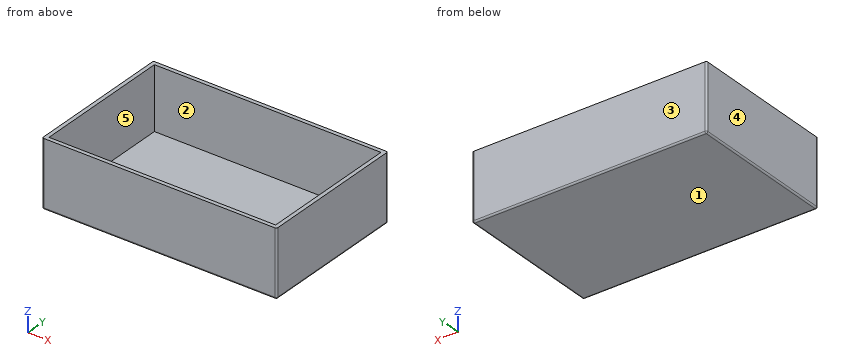
Autodesk Inventor part; units mm, degrees
ref_plane "YZ Plane" through (0, 0, 0) normal (1, 0, 0) x (0, 1, 0)
ref_plane "XZ Plane" through (0, 0, 0) normal (0, 1, 0) x (-1, 0, 0)
ref_plane "XY Plane" through (0, 0, 0) normal (0, 0, 1) x (1, 0, 0)
sketch "Sketch3" plane through (0, 0, 0) normal (0, 0, 1) x (1, 0, 0)
  line L0 (0, -133) -> (0, 133)
  line L1 (-210, 0) -> (210, 0)
  line L2 (-150, -95) -> (150, -95)
  line L3 (150, -95) -> (150, 95)
  line L4 (150, 95) -> (-150, 95)
  line L5 (-150, 95) -> (-150, -95)
  line L6 (-150, -95) -> (150, 95) construction
  line L7 (150, -95) -> (-150, 95) construction
  line L8 (-145, -90) -> (145, -90)
  line L9 (145, -90) -> (145, 90)
  line L10 (145, 90) -> (-145, 90)
  line L11 (-145, 90) -> (-145, -90)
  line L12 (-145, -90) -> (145, 90) construction
  line L13 (145, -90) -> (-145, 90) construction
  point P0 (0, 0)
  dimension "d0" = 300
  dimension "d1" = 190
  dimension "d2" = 290
  dimension "d3" = 180
extrude "Extrusion1" add sketch "Sketch3" along normal blind 85 contours L2 L5 L1 L11 L8 L0 | L0 L8 L9 L1 L3 L2 | L5 L4 L0 L10 L11 L1 | L1 L9 L10 L0 L4 L3
extrude "Extrusion2" add sketch "Sketch3" along normal blind 5 contours L8 L11 L1 L0 | L0 L1 L9 L8 | L1 L11 L10 L0 | L0 L10 L9 L1
fillet "Fillet1" radius 2 8 edges at (150, -95, 42.5) (150, 95, 42.5) (-150, 95, 42.5) (-150, -95, 42.5) (-150, 0, 0) (0, 95, 0) (0, -95, 0) (150, 0, 0)
equation "\"BendRadius\" = Thickness"
equation "\"BendReliefWidth\" = Thickness"
equation "\"BendReliefDepth\" = 0.5 * Thickness"
equation "\"CornerReliefSize\" = 4 * Thickness"
equation "\"MinimumRemnant\" = 2 * Thickness"
equation "\"TransitionRadius\" = BendRadius"
equation "\"JacobiRadiusSize\" = BendRadius"
equation "\"GapSize\" = Thickness"
properties part number "Batterybox"
The listing builds one solid part. Answer for the finished solid, in the listing's coordinates (mm). Face numbers are marked on the shaded views. A direction names the side the tool comes from. Coordinates: 2 decimals unless noted, no trailing zeros. Order: outer loops, then holes, each group sorted by start corner. A loop starts at its lowest first (then second) coordinate and runs counter-clockwise, first axis right, second up.
Q1. A cutting plane is placed at C-C, the plane y = -53.5. Write down the section's boundary in (x, z).
Q2. For a pull along Y with two mould halves and no side action, classify the marked faces 3, 4 and 5 as pulls with the +Y half, pulls with the -Y half, needs draft (parallel to the pull), parting line crosses it, or undercut.
Q3. Given P1, Ø1.5, axis at x = 94.5, y = 56.5, coming from the +Z side, flat-ended and moving along its own axis, determine where the tip first touches the part or whether it passes through.
Q4. A cutting plane is placed at A-A, the plane z = 10. Write down the section's boundary in (x, y), and give its area (3 significant figures).
Q5. A cutting plane is placed at B-B, the plane x = 88. Write down the section's boundary in (y, z), and give its area (3 significant figures).
Q6. Consider line 1 (Y direction, x = -124.5, z = 48.5); line 2 (X direction, y = 74.5, z = 23.5); line 3 (Z direction, x = -47, y = -26.5). Determine where each line is inside the solid, lowest interval first.
Q7. Which of the six approach directions +Z, -Z, +X, -X, +Y, -Y give full straight-line access (tool end or side, diameter ignored) to the marked faces 1 and 2?
Answers follow:
1. outline: (-150, 2) arc R2 ccw to (-148, 0) - (148, 0) arc R2 ccw to (150, 2) - (150, 85) - (145, 85) - (145, 5) - (-145, 5) - (-145, 85) - (-150, 85) - close
2. face 3: pulls with the +Y half
2. face 4: needs draft
2. face 5: undercut
3. P1: stops at z = 5
4. outline: (-150, -93) arc R2 ccw to (-148, -95) - (148, -95) arc R2 ccw to (150, -93) - (150, 93) arc R2 ccw to (148, 95) - (-148, 95) arc R2 ccw to (-150, 93) - close; hole (-145, -90) - (145, -90) - (145, 90) - (-145, 90) - close
4. area: 4,800 mm2
5. outline: (-95, 2) arc R2 ccw to (-93, 0) - (93, 0) arc R2 ccw to (95, 2) - (95, 85) - (90, 85) - (90, 5) - (-90, 5) - (-90, 85) - (-95, 85) - close
5. area: 1,750 mm2
6. line 1: y = -95 to -90, 90 to 95
6. line 2: x = -150 to -145, 145 to 150
6. line 3: z = 0 to 5
7. face 1: -Z, +X, -X, +Y, -Y
7. face 2: +Z
